from build123d import *

# Parameters (mm, degrees)
CUT_EXTRUDE1_DEPTH      = 54.63402325
CUT_EXTRUDE1_DEPTH_BACK = 54.63402325
SKETCH2_R               = 1.3
F7F_R                   = 0.5
CUT_EXTRUDE2_DEPTH      = 54.634023349
CUT_EXTRUDE2_DEPTH_BACK = 54.634023349
SKETCH3_W               = 6.35
SKETCH3_H               = 30.7
FILLET1_R               = 0.5


with BuildPart() as part:
    # Sketch1 → Revolve1 (revolve)
    with BuildSketch(Plane.YZ, mode=Mode.PRIVATE) as revolve1_sk:
        Polygon((0, 0), (4.815, 0), (4.815, -2.4), (3.175, -2.4), (3.175, -53.2), (0, -53.2), align=None)
    revolve(revolve1_sk.sketch.rotate(Axis((0, 0, -335.576810525), (0, 0, 1)), 90), axis=Axis((0, 0, -335.576810525), (0, 0, 1)))

    # Sketch2 → Cut-Extrude1 (cut, two sides: drawn at the far end of the back side and taken through both)
    with BuildSketch(Plane.YZ.offset(-CUT_EXTRUDE1_DEPTH_BACK)):
        with Locations(Location((0, -47.7, 0), (0, 0, 270.000000002))):
            Circle(SKETCH2_R)
        with Locations(Location((0, -42.1, 0), (0, 0, 270.000000002))):
            Circle(SKETCH2_R)
        with Locations(Location((0, -25.3, 0), (0, 0, 270.000000002))):
            Circle(SKETCH2_R)
        with Locations(Location((0, -30.9, 0), (0, 0, 270.000000002))):
            Circle(SKETCH2_R)
        with Locations(Location((0, -36.5, 0), (0, 0, 270.000000002))):
            Circle(SKETCH2_R)
        with Locations(Location((0, -19.7, 0), (0, 0, 270.000000002))):
            Circle(SKETCH2_R)
    extrude(amount=CUT_EXTRUDE1_DEPTH + CUT_EXTRUDE1_DEPTH_BACK, mode=Mode.SUBTRACT)

    # f7f
    f7f_edges = [part.edges().sort_by_distance(p)[0] for p in [
        (4.815, 0, -2.4),
        (4.815, 0, 0),
    ]]
    fillet(f7f_edges, radius=F7F_R)

    # Sketch3 → Cut-Extrude2 (cut, two sides: drawn at the far end of the back side and taken through both)
    with BuildSketch(Plane.YZ.offset(-CUT_EXTRUDE2_DEPTH_BACK)):
        with Locations((0, -37.85)):
            Rectangle(SKETCH3_W, SKETCH3_H)
    extrude(amount=CUT_EXTRUDE2_DEPTH + CUT_EXTRUDE2_DEPTH_BACK, mode=Mode.SUBTRACT)

    # Fillet1
    fillet1_edges = [part.edges().sort_by_distance(p)[0] for p in [
        (3.175, 0, -22.5),
    ]]
    fillet(fillet1_edges, radius=FILLET1_R)


solid = part.part
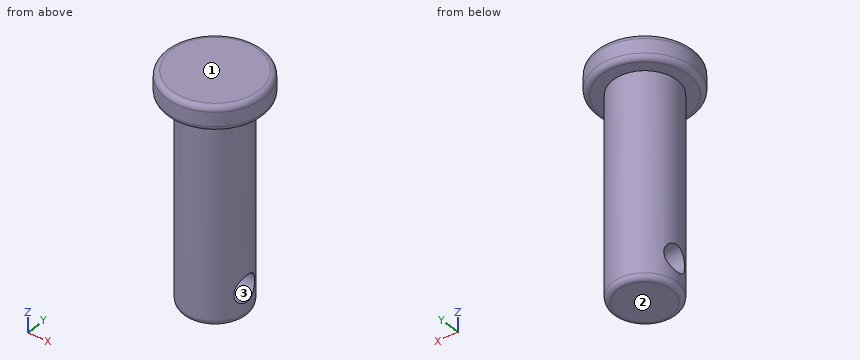
Here's how the part is built. I have some questions about the finished solid (model axes, mm). Face numbers are marked on the shaded views. Round coordinates to 2 decimals unless told otherwise and drop trailing zeros. Loops run counter-clockwise (first coordinate to the right, second up) from the corner with the lowest first, then second, coordinate; pieces in that order, holes last.
1. If we section it at B-B on z = -6.75: Write out the boundary of the cut face in (x, y) (3 decimals), plus the area to 3 significant figures.
Answer list:
outline: circle Ø6.35 at (0, 0)
area: 31.7 mm2
2. If I drill on line 1 along Y through (x, z) = (0, -19.7) (3 decimals); line 2 along Z through (x, y) = (-1, -0.5); line 3 along Z through (x, y) = (2.25, -3.5), over which ranges is the centre line in solid material (lowest first)?
Answer list:
line 1: y = -3.175 to -1.3, 1.3 to 3.175
line 2: z = -22.5 to -20.9, -18.5 to 0
line 3: z = -2.4 to 0
3. For P1, Ø5, axis at y = -1.5, z = -10.5, coming from the -X side (3 decimals); P2, Ø4, axis at x = 1, z = -19.5, coming from the +Y side (3 decimals); P3, Ø1, axis at y = -3, z = -16.5, coming from the +X side, each with a flat end and sliding along its axis, tell me the tip position at first contact or that it passes through.
Answer list:
P1: stops at x = -3.175
P2: stops at y = 3.175
P3: stops at x = 1.96
4. If we section it at C-C on z = -19.7: Write out the boundary of the cut face in (x, y) (3 decimals).
Answer list:
outline: (-2.897, -1.3) arc R3.175 ccw to (2.897, -1.3) - close; (-2.897, 1.3) - (2.897, 1.3) arc R3.175 ccw to start
5. If we section it at A-A on x = 0: Write out the boundary of the cut face in (y, z) (3 decimals), plus the area to 3 significant figures.
Answer list:
outline: (-4.815, -1.9) arc R0.5 ccw to (-4.315, -2.4) - (-3.175, -2.4) - (-3.175, -22) arc R0.5 ccw to (-2.675, -22.5) - (2.675, -22.5) arc R0.5 ccw to (3.175, -22) - (3.175, -2.4) - (4.315, -2.4) arc R0.5 ccw to (4.815, -1.9) - (4.815, -0.5) arc R0.5 ccw to (4.315, 0) - (-4.315, 0) arc R0.5 ccw to (-4.815, -0.5) - close; hole circle Ø2.6 at (0, -19.7)
area: 145 mm2
6. We'd pull the mould along Z, two halves only. Please class the marked faces 1, 2 and 3: +Z half, -Z half, draft (parallel to the pull), parting line (faces both ways), or undercut.
Answer list:
face 1: +Z half
face 2: -Z half
face 3: undercut
